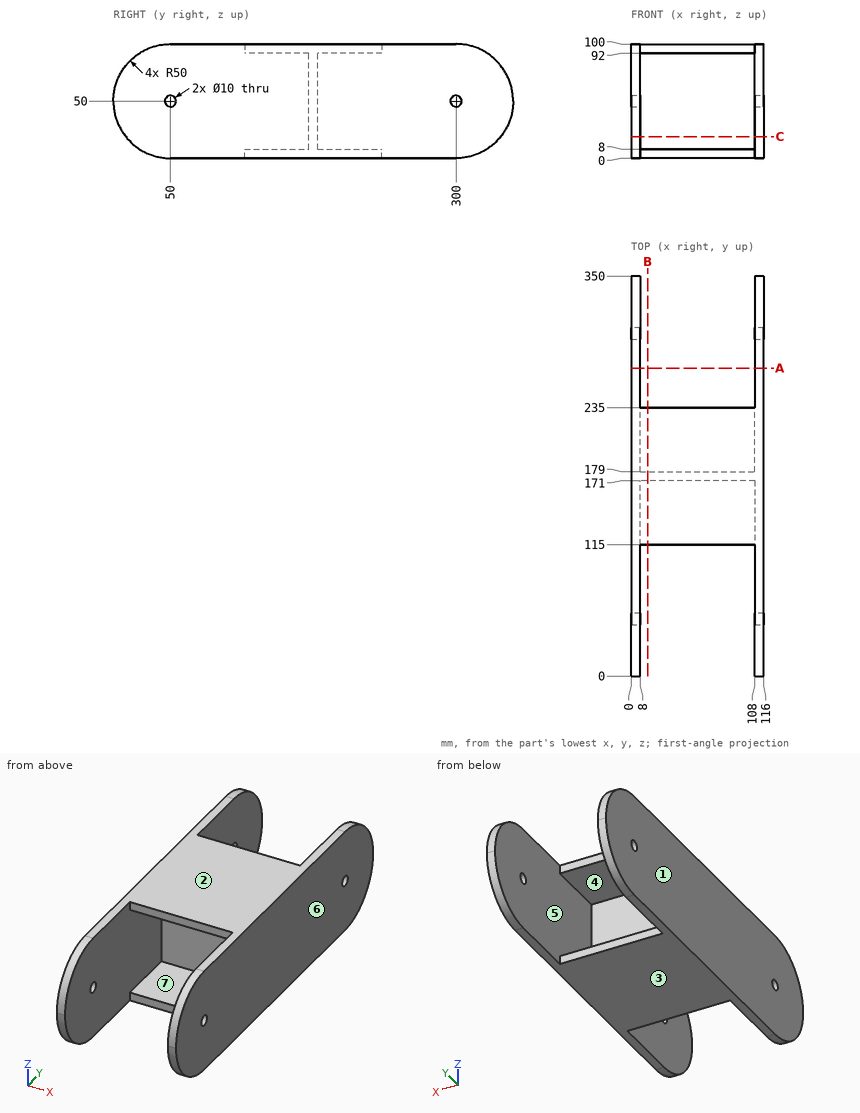
Design review of the part shown in the three views and the two pictorial views. Dimensions are in mm from the part's minimum x, y and z. A direction names the side the tool comes from. Round coordinates to 2 decimals unless told otherwise and drop trailing zeros. Write each loop counter-clockwise with the first axis right and the second up, starting at its lowest first coordinate (ties: lowest second). Pieces come first, ordered by that corner, then holes.
1) Take a section at C-C on z = 19. Give the boundary of the cut face in (x, y).
Answer below:
outline: (0, 10.77) - (8, 10.77) - (8, 171) - (108, 171) - (108, 10.77) - (116, 10.77) - (116, 339.23) - (108, 339.23) - (108, 179) - (8, 179) - (8, 339.23) - (0, 339.23) - close
2) Take a section at B-B on x = 14.5. Give the boundary of the cut face in (y, z), then the cut area to 3 significant figures.
Answer below:
outline: (115, 0) - (235, 0) - (235, 8) - (179, 8) - (179, 92) - (235, 92) - (235, 100) - (115, 100) - (115, 92) - (171, 92) - (171, 8) - (115, 8) - close
area: 2,590 mm2
3) Insertion check: pin 1 Ø6.5 at (x, z) = (35, 96.5) entering from -Y; pin 2 Ø9 at (x, z) = (49.5, 97.5) entering from +Y; pin 3 Ø1.5 at (x, z) = (12, 77) entering from +Y; pin 4 Ø6 at (y, z) = (50, 50) entering from +X. Each pin has a flat end and moves straight along its axis. Give the tip position at first contact, or say it passes through.
Answer below:
pin 1: stops at y = 115
pin 2: stops at y = 235
pin 3: stops at y = 179
pin 4: passes through
4) Mouldability with a two-part tool opening along Z and no side actions: class the marked faces 1, 2, 3 and 4 as +Z half, -Z half, draft (parallel to the pull), parting line (faces both ways), or undercut.
Answer below:
face 1: draft
face 2: +Z half
face 3: -Z half
face 4: undercut
5) For line 1 along Z through (x, y) = (110.5, 300); line 2 along X through (y, z) = (213, 28); line 3 along Y through (x, z) = (60.5, 77.5), list the stretches that pass through material, from the lowest coordinate up.
Answer below:
line 1: z = 0 to 45, 55 to 100
line 2: x = 0 to 8, 108 to 116
line 3: y = 171 to 179
6) Machinability: for the marked faces 5, 6 and 7, which of the approach directions +Z, -Z, +X, -X, +Y, -Y give a long, thin tool a straight path to every point of the face, cutting with its end or side? Answer none if there is none.
Answer below:
face 5: +Y
face 6: +Z, -Z, +X, +Y, -Y
face 7: -Y
7) Take a section at A-A on y = 269.5. Give the boundary of the cut face in (x, z), then the cut area to 3 significant figures.
Answer below:
outline: (0, 0) - (8, 0) - (8, 100) - (0, 100) - close; (108, 0) - (116, 0) - (116, 100) - (108, 100) - close
area: 1,600 mm2
